Part model, mm, in its own coordinate system. Coordinates: 2 decimals unless noted, no trailing zeros. Loops run counter-clockwise (first coordinate to the right, second up) from the corner with the lowest first, then second, coordinate; pieces in that order, holes last. Notation, with made-up numbers: (17, -34) -> (28, -34) arc R13 cw to (28, -16) -> close; hole circle Ø8 at (53, 67.25). An arc over 180 degrees is marked (long way). Use one line per item in the form item = value. Start each with the question number.
(1) Band-saw the part on C-C on y = -0.7. Give the cut face in (x, z), then the cut area to 3 significant figures.
(2) Band-saw the part on D-D on x = -7. Give the cut face in (y, z), then the cut area to 3 significant figures.
(3) Pin check, flat tips, straight feed: P1, Ø6, axis at x = -9, z = 16.5, coming from the +Y side; P2, Ø4, axis at x = -9, z = 42.5, coming from the +Y side. Stop position of each tip, or through.
(4) Drill centre lines: L1, parallel to Z at x = -9, y = -1.05; L2, parallel to Z at x = -7.5, y = -0.5; L3, parallel to X at y = -0.7, z = 8. Where is each one in solid material? Low to high. Write a range as [from, to].
(5) Band-saw the part on A-A on x = -10.5. Give the cut face in (y, z), then the cut area to 3 significant figures.
(6) Band-saw the part on B-B on z = 42.5. Give the cut face in (x, y).
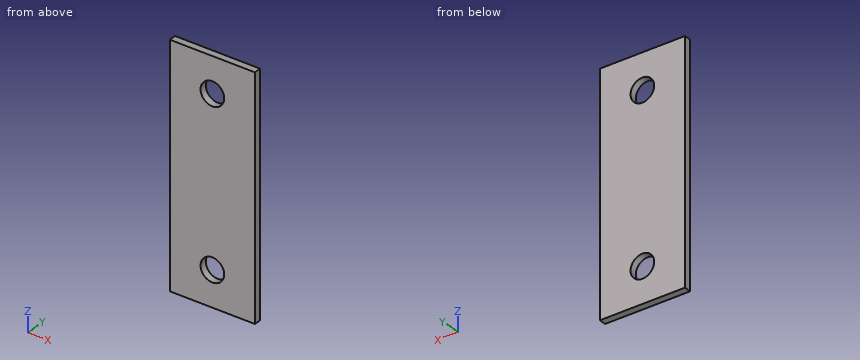
```python
from build123d import *

# Parameters (mm, degrees)
F0_W     = 18
F0_H     = 50
F0_R     = 2.5
F1_DEPTH = 1.5


# Not quite as in the source:
# - a feature names something its author has since deleted; it is built from what else it names


with BuildPart() as f1:
    # F0 (on Front) → F1 (new body)
    with BuildSketch(Plane.XZ):
        with Locations((-9, 25)):
            Rectangle(F0_W, F0_H)
        with Locations((-9, 7.5)):
            Circle(F0_R, mode=Mode.SUBTRACT)
        with Locations((-9, 42.5)):
            Circle(F0_R, mode=Mode.SUBTRACT)
    extrude(amount=F1_DEPTH)


solid = f1.part
```
A:
q1.outline = (-18, 0) -> (0, 0) -> (0, 50) -> (-18, 50) -> close; hole circle Ø5 at (-9, 7.5); hole circle Ø5 at (-9, 42.5)
q1.area = 861 mm²
q2.outline = (-1.5, 0) -> (0, 0) -> (0, 6) -> (-1.5, 6) -> close; (-1.5, 9) -> (0, 9) -> (0, 41) -> (-1.5, 41) -> close; (-1.5, 44) -> (0, 44) -> (0, 50) -> (-1.5, 50) -> close
q2.area = 66.0 mm²
q3.P1 = 0
q3.P2 = through
q4.L1 = [0, 5], [10, 40], [45, 50]
q4.L2 = [0, 5.5], [9.5, 40.5], [44.5, 50]
q4.L3 = [-18, -11.45], [-6.55, 0]
q5.outline = (-1.5, 0) -> (0, 0) -> (0, 5.5) -> (-1.5, 5.5) -> close; (-1.5, 9.5) -> (0, 9.5) -> (0, 40.5) -> (-1.5, 40.5) -> close; (-1.5, 44.5) -> (0, 44.5) -> (0, 50) -> (-1.5, 50) -> close
q5.area = 63.0 mm²
q6.outline = (-18, -1.5) -> (-11.5, -1.5) -> (-11.5, 0) -> (-18, 0) -> close; (-6.5, -1.5) -> (0, -1.5) -> (0, 0) -> (-6.5, 0) -> close
